Read the model definition and answer for the solid it produces. Units are mm, in the model's axes. A direction names the side the tool comes from. Round coordinates to 2 decimals unless told otherwise and drop trailing zeros. Loops run counter-clockwise (first coordinate to the right, second up) from the corner with the lowest first, then second, coordinate; pieces in that order, holes last. Notation, with made-up numbers: (29, 6) -> (77, 6) arc R12 ccw to (77, 11) -> close; hole circle Ø4 at (-33, 62.25). An arc over 180 degrees is marked (long way). Put each result on its own line as item: value.
from build123d import *

# Parameters (mm, degrees)
SKETCH1_W                       = 240
SKETCH1_H                       = 30
BOSS_EXTRUDE2_DEPTH             = 120
BOSS_EXTRUDE3_REACH             = 166.118
BOSS_EXTRUDE3_DIRECTION_2_REACH = 166.118
SKETCH7_W                       = 50
SKETCH7_H                       = 70
CUT_EXTRUDE1_DEPTH              = 250
SKETCH8_R                       = 10
SKETCH8_R_2                     = 15
BOSS_EXTRUDE4_DEPTH             = 30
FILLET1_R                       = 5


with BuildPart() as part:
    # Sketch1 → Boss-Extrude2 (new body, symmetric)
    with BuildSketch(Plane.XY):
        Rectangle(SKETCH1_W, SKETCH1_H)
    extrude(amount=BOSS_EXTRUDE2_DEPTH, both=True)

    # Boss-Extrude3: up to this face of the body (flat: up to its plane)
    boss_extrude3_end = Plane(part.part.faces().sort_by_distance((-120, 0, 0))[0])
    # Sketch6 → Boss-Extrude3 (add, up to the picked face)
    with BuildSketch(Plane(origin=(0, 0, 0), x_dir=(-0.503871026, 0, -0.863778901), z_dir=(0.863778901, 0, -0.503871026)), mode=Mode.PRIVATE) as boss_extrude3_sk1:
        with BuildLine():
            Line((35, 0), (35, 50))
            ThreePointArc((35, 50), (0, 85), (-35, 50))
            Line((-35, 50), (-35, 0))
            Line((-35, 0), (35, 0))
        make_face()
        Polygon((23.094010768, 50), (11.547005384, 70), (-11.547005384, 70), (-23.094010768, 50), (-11.547005384, 30), (11.547005384, 30), align=None, mode=Mode.SUBTRACT)
    boss_extrude3_tool1 = split(extrude(boss_extrude3_sk1.sketch, amount=-BOSS_EXTRUDE3_REACH, mode=Mode.PRIVATE), bisect_by=boss_extrude3_end, keep=Keep.BOTH, mode=Mode.PRIVATE)
    add(boss_extrude3_tool1.solids().sort_by_distance((17.080655, 25, 29.281124))[0])

    # Boss-Extrude3 direction 2: up to this face of the body (flat: up to its plane)
    boss_extrude3_direction_2_end = Plane(part.part.faces().sort_by_distance((120, 0, 0))[0])
    # Sketch6 → Boss-Extrude3 direction 2 (add, up to the picked face)
    with BuildSketch(Plane(origin=(0, 0, 0), x_dir=(-0.503871026, 0, -0.863778901), z_dir=(0.863778901, 0, -0.503871026)), mode=Mode.PRIVATE) as boss_extrude3_direction_2_sk1:
        with BuildLine():
            Line((35, 0), (35, 50))
            ThreePointArc((35, 50), (0, 85), (-35, 50))
            Line((-35, 50), (-35, 0))
            Line((-35, 0), (35, 0))
        make_face()
        Polygon((23.094010768, 50), (11.547005384, 70), (-11.547005384, 70), (-23.094010768, 50), (-11.547005384, 30), (11.547005384, 30), align=None, mode=Mode.SUBTRACT)
    boss_extrude3_direction_2_tool1 = split(extrude(boss_extrude3_direction_2_sk1.sketch, amount=BOSS_EXTRUDE3_DIRECTION_2_REACH, mode=Mode.PRIVATE), bisect_by=boss_extrude3_direction_2_end, keep=Keep.BOTH, mode=Mode.PRIVATE)
    add(boss_extrude3_direction_2_tool1.solids().sort_by_distance((17.080655, 25, 29.281124))[0])

    # Sketch7 → Cut-Extrude1 (cut)
    with BuildSketch(Plane(origin=(0, 0, -70), x_dir=(-1, 0, 0), z_dir=(0, 0, -1))):
        with Locations((0, 50)):
            Rectangle(SKETCH7_W, SKETCH7_H)
    extrude(amount=-CUT_EXTRUDE1_DEPTH, mode=Mode.SUBTRACT)

    # Sketch8 → Boss-Extrude4 (add)
    with BuildSketch(Plane(origin=(0, 15, 0), x_dir=(1, 0, 0), z_dir=(0, 1, 0))):
        with Locations((-90, 60)):
            Circle(SKETCH8_R)
        with Locations((65, -75)):
            Circle(SKETCH8_R_2)
    extrude(amount=BOSS_EXTRUDE4_DEPTH)

    # Fillet1
    fillet1_edges = [part.edges().sort_by_distance(p)[0] for p in [
        (50, 45, 75),
        (-100, 45, -60),
    ]]
    fillet(fillet1_edges, radius=FILLET1_R)


solid = part.part
Item 1: The part is cut by section A-A (y = 78.5). Determine the outline of the cut face in (x, z), then the cut area to 3 significant figures.
Derived:
outline: (-120, 46.48) -> (-25, -8.94) -> (-25, 38.1) -> (-120, 93.52) -> close; (25, -38.1) -> (120, -93.52) -> (120, -46.48) -> (25, 8.94) -> close
area: 8,940 mm^2
Item 2: Find the intervals of material crossed by line 1 along Y through (x, z) = (29, 102.5); line 2 along X through (y, z) = (77, -10.5); line 3 along X through (y, z) = (44, -105), in increasing order.
Derived:
line 1: y = -15 to 15
line 2: x = -26.2 to -25, 25 to 62.2
line 3: x = 110.54 to 120
Item 3: For a pull along X with two mould halves and no side action, classify faces 1 (the flat face through (-73.165, 39.86, 22.721)), 2 (the flat face through (-2, 0, -120)), 3 (the flat face through (-73.165, 32.255, 2.16)) as pulls with the +X half, pulls with the -X half, needs draft (parallel to the pull), parting line crosses it, or undercut.
Derived:
face 1: undercut
face 2: needs draft
face 3: pulls with the -X half
Item 4: Which of the six approach directions +Z, -Z, +X, -X, +Y, -Y give full straight-line access (tool end or side, diameter ignored) to faces 4 (the flat face through (65, 45, 75)), 5 (the flat face through (-73.17, 32.74, 83.2)), 6 (the flat face through (72, 30, -42)), 7 (the cylindrical face through (61.748, 27.325, 89.643))?
Derived:
face 4: +Z, +X, +Y
face 5: +Z, +Y
face 6: none
face 7: +Y
Item 5: The part is cut by section B-B (y = 53.5). Determine the outline of the cut face in (x, z), then the cut area to 3 significant figures.
Derived:
outline: (-120, 29.68) -> (-25, -25.73) -> (-25, -9.81) -> (-120, 45.6) -> close; (-120, 94.4) -> (-25, 38.98) -> (-25, 54.9) -> (-120, 110.32) -> close; (25, -54.9) -> (120, -110.32) -> (120, -94.4) -> (25, -38.98) -> close; (25, 9.81) -> (120, -45.6) -> (120, -29.68) -> (25, 25.73) -> close
area: 6,050 mm^2
Item 6: Flat-ended cylindrical pins translate along their axes: pin 1 Ø12 at (x, y) = (-67, 68) entering from -Z; pin 2 Ø2 at (x, z) = (-29.5, 0) entering from +Y; pin 3 Ø16 at (x, z) = (65.5, 75.5) entering from +Y. Find the tip coordinate at first contact, or state that the pin passes through.
Derived:
pin 1: stops at z = -0.66
pin 2: stops at y = 82.14
pin 3: stops at y = 45
